Build history of the part. All positions in model axes, mm. Face numbers are marked on the shaded views. A direction names the side the tool comes from. Give positions to 0.01 mm unless a question says otherwise; leave off trailing zeros. Order: outer loops, then holes, each group sorted by start corner. A loop starts at its lowest first (then second) coordinate and runs counter-clockwise, first axis right, second up. Notation, with made-up numbers: (-31, 64) -> (-18, 64) arc R15 cw to (-18, 74) -> close; hole circle Ø2 at (-36, 80.5). An arc over 180 degrees is marked (long way). Use a Markdown table: item, result. Add a question column.
```python
from build123d import *

# Parameters (mm, degrees)
F0_R     = 7.62
F1_DEPTH = 177.8
F2_R     = 13.3961088479
F3_DEPTH = 33.02
F4_R     = 8.9999575192
F5_DEPTH = 83.312


with BuildPart() as f1:
    # F0 (on Front) → F1 (new body)
    with BuildSketch(Plane.XZ):
        Circle(F0_R)
    extrude(amount=F1_DEPTH)

    # F2 (on Right) → F3 (join, symmetric)
    with BuildSketch(Plane.YZ):
        with Locations((-187.3978376389, 0)):
            Circle(F2_R)
    extrude(amount=F3_DEPTH, both=True)

    # F4 (on face) → F5 (cut)
    with BuildSketch(Plane.YZ.offset(33.02)):
        with Locations((-187.3978376389, 0)):
            Circle(F4_R)
    extrude(amount=-F5_DEPTH, mode=Mode.SUBTRACT)


solid = f1.part
```
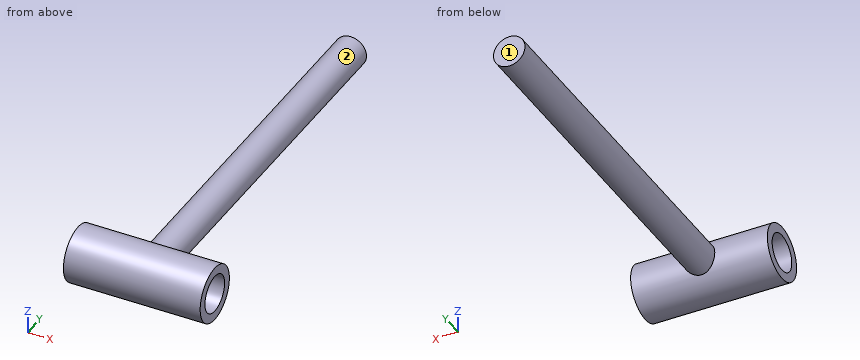
(1) Band-saw the part on A-A on z = 0. Give the cut face in (x, y), plus the area to 3 significant figures.
(2) Band-saw the part on D-D on z = 10.75. Give the cut face in (x, y).
(3) Pin check, flat tips, straight feed: pin 1 Ø3 at (x, y) = (21, -176) entering from -Z; pin 2 Ø12 at (x, z) = (3.5, -8) entering from +Y; pin 3 Ø10 at (x, z) = (-22, -0.5) entering from +Y; pin 4 Ø4 at (y, z) = (-166, 0.5) entering from +X. Stop position of each tip, or through.
(4) Band-saw the part on B-B on x = 0. Give the cut face in (y, z), plus the area to 3 significant figures.
(5) Band-saw the part on C-C on y = -147.5. Give the cut face in (x, z), plus the area to 3 significant figures.
(6) Wall check: probe 1 along Y at (x, z) = (29, 0.5); probe 2 along Y at (x, z) = (14.5, -3.75); probe 3 along Z at (x, y) = (-3.5, -144). Give the ranges that are in metal, low to high.
(7) Tool access for the marked faces 1 and 2: list every direction of +Z, -Z, +X, -X, +Y, -Y with a clear straight run to the whole face (end or side of a thin tool).
Response:
| question | item | result |
|---|---|---|
| 1 | outline | (-33.02, -200.79) -> (33.02, -200.79) -> (33.02, -196.4) -> (-33.02, -196.4) -> close; (-33.02, -178.4) -> (33.02, -178.4) -> (33.02, -174) -> (7.62, -174) -> (7.62, 0) -> (-7.62, 0) -> (-7.62, -174) -> (-33.02, -174) -> close |
| 1 | area | 3,230 mm² |
| 2 | outline | (-33.02, -195.39) -> (33.02, -195.39) -> (33.02, -179.4) -> (-33.02, -179.4) -> close |
| 3 | pin 1 | stops at z = -9.03 |
| 3 | pin 2 | stops at y = 0 |
| 3 | pin 3 | stops at y = -174 |
| 3 | pin 4 | stops at x = 7.62 |
| 4 | outline | (-176.38, -7.62) -> (0, -7.62) -> (0, 7.62) -> (-176.38, 7.62) arc R13.4 ccw (long way) to start; hole circle Ø18 at (-187.4, 0) |
| 4 | area | 2,970 mm² |
| 5 | outline | circle Ø15.24 at (0, 0) |
| 5 | area | 182 mm² |
| 6 | probe 1 | y = -200.78 to -196.38, -178.41 to -174.01 |
| 6 | probe 2 | y = -200.26 to -195.58, -179.22 to -174.54 |
| 6 | probe 3 | z = -6.77 to 6.77 |
| 7 | face 1 | +Z, -Z, +X, -X, +Y |
| 7 | face 2 | +Y |
